Verification items for the finished model (mm, model axes). A direction names the side the tool comes from. Coordinates: 2 decimals unless noted, no trailing zeros. Order: outer loops, then holes, each group sorted by start corner. A loop starts at its lowest first (then second) coordinate and runs counter-clockwise, first axis right, second up. Notation, with made-up numbers: (32, 50) - (67, 50) arc R14 ccw to (67, 68) - close; hole circle Ø10 at (89.25, 12). An arc over 180 degrees is marked (long way). Answer as CSV lines item,"result". Start each with the question number.
1. Section check B-B (y = -1.5). Record the cut outline in (x, z), and give its area (3 significant figures).
2. Section check D-D (z = 14.25). Record the cut outline in (x, y).
3. Set-up check for faces 1 (the cylindrical face through (4.23, -6.79, 3.94)), 2 (the flat face through (7, 0, 6)), 3 (the cylindrical face through (0, 9, 11)), 4 (the flat face through (-7, 0, 6)): record each of +Z, -Z, +X, -X, +Y, -Y from which the full face is reachable in a straight line by a thin tool's end or side.
4. Section check C-C (x = 9.75). Record the cut outline in (y, z), and give its area (3 significant figures).
5. Go/stop test with flat-tipped pins: pin 1 (12 mm diameter, centred on x = 8, z = 2.5, fed in from -Y); pin 2 (2 mm diameter, centred on y = -6.5, z = 15.5, fed in from -X); pin 3 (1.5 mm diameter, centred on x = 4, y = -8, fed in from -Z). Record where each tip stops, or that it passes through.
6. Section check A-A (z = 7.5). Record the cut outline in (x, y), and give its area (3 significant figures).
7. Material ranges on L1, parallel to X at y = -3.5, z = 1; L2, parallel to Z at x = -7.25, y = -5.25; L3, parallel to X at y = 4.5, z = 14.5, recorded low to high. Write a range as [from, to].
from build123d import *

# Parameters (mm, degrees)
SKIZZE1_R                       = 8
AUFSATZ_LINEAR_AUSTRAGEN1_DEPTH = 8
SKIZZE2_R                       = 9
AUFSATZ_LINEAR_AUSTRAGEN2_DEPTH = 5
AUFSATZ_LINEAR_AUSTRAGEN3_DEPTH = 8
SKIZZE4_W                       = 3
SKIZZE4_H                       = 19.049807725
SCHNITT_LINEAR_AUSTRAGEN1_DEPTH = 13
VERRUNDUNG1_R                   = 1
SKIZZE5_W                       = 1
SKIZZE5_H                       = 3.315694734
AUFSATZ_LINEAR_AUSTRAGEN4_DEPTH = 13


with BuildPart() as part:
    # Skizze1 → Aufsatz-Linear austragen1 (new body)
    with BuildSketch(Plane.XY):
        Circle(SKIZZE1_R)
    extrude(amount=AUFSATZ_LINEAR_AUSTRAGEN1_DEPTH)

    # Skizze2 → Aufsatz-Linear austragen2 (add)
    with BuildSketch(Plane.XY.offset(8)):
        Circle(SKIZZE2_R)
    extrude(amount=AUFSATZ_LINEAR_AUSTRAGEN2_DEPTH)

    # Skizze3 → Aufsatz-Linear austragen3 (add)
    with BuildSketch(Plane.XY.offset(13)):
        Polygon((11.995271167, 0), (5.997635583, 10.388209556), (-5.997635583, 10.388209556), (-11.995271167, 0), (-5.997635583, -10.388209556), (5.997635583, -10.388209556), align=None)
    extrude(amount=AUFSATZ_LINEAR_AUSTRAGEN3_DEPTH)

    # Skizze4 → Schnitt-Linear austragen1 (cut)
    with BuildSketch(Plane(origin=(0, 0, 0), x_dir=(-1, 0, 0), z_dir=(0, 0, -1))):
        with Locations((-8.5, -0.043792661)):
            Rectangle(SKIZZE4_W, SKIZZE4_H)
        with Locations((8.5, -0.043792661)):
            Rectangle(SKIZZE4_W, SKIZZE4_H)
    extrude(amount=-SCHNITT_LINEAR_AUSTRAGEN1_DEPTH, mode=Mode.SUBTRACT)

    # Verrundung1
    verrundung1_edges = [part.edges().sort_by_distance(p)[0] for p in [
        (0, -9, 8),
        (0, 9, 8),
    ]]
    fillet(verrundung1_edges, radius=VERRUNDUNG1_R - 0.0001)  # a hair under: the kernel refuses the full size

    # Skizze5 → Aufsatz-Linear austragen4 (add)
    with BuildSketch(Plane(origin=(0, 0, 13), x_dir=(-1, 0, 0), z_dir=(0, 0, -1))):
        with Locations((0, -8.730362189)):
            Rectangle(SKIZZE5_W, SKIZZE5_H)
    extrude(amount=AUFSATZ_LINEAR_AUSTRAGEN4_DEPTH)


solid = part.part
Evaluation:
1,outline,"(-11.13, 13) - (-7, 13) - (-7, 0) - (7, 0) - (7, 13) - (11.13, 13) - (11.13, 21) - (-11.13, 21) - close"
1,area,"360 mm²"
2,outline,"(-12, 0) - (-6, -10.39) - (6, -10.39) - (12, 0) - (6, 10.39) - (-6, 10.39) - close"
3,face 1,"-Z, +X, -Y"
3,face 2,"-Z, +X, +Y, -Y"
3,face 3,"-Z, +Y"
3,face 4,"-Z, -X, +Y, -Y"
4,outline,"(-3.89, 13) - (3.89, 13) - (3.89, 21) - (-3.89, 21) - close"
4,area,"62.2 mm²"
5,pin 1,"stops at y = -7.75"
5,pin 2,"stops at x = -8.82"
5,pin 3,"stops at z = 8.02"
6,outline,"(-7, -3.87) arc R8 ccw to (-0.5, -7.98) - (-0.5, -10.39) - (0.5, -10.39) - (0.5, -7.98) arc R8 ccw to (7, -3.87) - (7, 3.87) arc R8 ccw to (-7, 3.87) - close"
6,area,"193 mm²"
7,L1,"x = [-7, 7]"
7,L2,"z = [13, 21]"
7,L3,"x = [-9.4, 9.4]"
